Check sheet for the modelled part. Datum: model origin and axes. Units: mm. Face numbers are marked on the shaded views. A direction names the side the tool comes from. Round coordinates to 2 decimals unless told otherwise and drop trailing zeros. Loops run counter-clockwise (first coordinate to the right, second up) from the corner with the lowest first, then second, coordinate; pieces in that order, holes last. Notation, with made-up numbers: M 53,64.5 L 86,64.5 A24 ccw 86,79.5 Z; hole C 28,60 d8. An arc over 180 degrees is marked long. Write item = value, one per line. Start each with the question number.
(1) Cross-section at D-D on y = 0. Record the boundary of the cut face in (x, z), plus the area to 3 significant figures.
(2) Set-up check for the marked faces 4, 5 and 6: record each of +Z, -Z, +X, -X, +Y, -Y from which the full face is reachable in a straight line by a thin tool's end or side.
(3) Mould release check, pull along Z, two halves, no side actions. Record for the marked faces 1, 2 and 3: pulls with the +Z half, pulls with the -Z half, needs draft (parallel to the pull), parting line crosses it, or undercut.
(4) Cross-section at A-A on z = 10.75. Record the boundary of the cut face in (x, y).
(5) Cross-section at C-C on y = 6. Record the boundary of the cut face in (x, z).
(6) Scan lines: L1, parallel to Y at x = 1.45, z = -10.75; L2, parallel to X at y = -2.75, z = 13; L3, parallel to Y at x = 1, z = 0. Record each from-to range of solid material in increasing order. Write a range as from..to.
(7) Cross-section at B-B on x = 2.5. Record the boundary of the cut face in (y, z), plus the area to 3 significant figures.
(8) Go/stop test with flat-tipped pins: P1, Ø1, axis at x = 1, y = 3, coming from the +Z side; P2, Ø0.6, axis at x = 2, y = 3, coming from the -Z side; P3, Ø2, axis at y = 0, z = 10.75, coming from the +X side; P4, Ø4, axis at y = 0, z = -10.75, coming from the +X side. Record where each tip stops, or that it passes through.
from build123d import *

# Parameters (mm, degrees)
SKETCH1_W           = 40
SKETCH1_H           = 15
BOSS_EXTRUDE1_DEPTH = 3
SKETCH2_R           = 1.25
CUT_EXTRUDE1_DEPTH  = 5
FILLET1_R           = 8
BOSS_EXTRUDE2_START = 4
BOSS_EXTRUDE2_DEPTH = 4
FILLET2_R           = 4


with BuildPart() as part:
    # Sketch1 → Boss-Extrude1 (new body)
    with BuildSketch(Plane(origin=(0, 0, 0), x_dir=(0, 0, -1), z_dir=(1, 0, 0))):
        Rectangle(SKETCH1_W, SKETCH1_H)
    extrude(amount=BOSS_EXTRUDE1_DEPTH)

    # Sketch2 → Cut-Extrude1 (cut)
    with BuildSketch(Plane(origin=(3, 0, 0), x_dir=(0, 0, -1), z_dir=(1, 0, 0))):
        with Locations((-10.75, 0)):
            Circle(SKETCH2_R)
        with BuildLine():
            Line((-3, 2.25), (-3, 7.5))
            Line((-3, 7.5), (3, 7.5))
            Line((3, 7.5), (3, 2.25))
            ThreePointArc((3, 2.25), (0, -0.75), (-3, 2.25))
        make_face()
    cut_extrude1 = extrude(amount=-CUT_EXTRUDE1_DEPTH, mode=Mode.SUBTRACT)

    # Mirror1: Cut-Extrude1 across plane
    add(cut_extrude1.mirror(Plane.XY), mode=Mode.SUBTRACT)

    # Fillet1
    fillet1_edges = [part.edges().sort_by_distance(p)[0] for p in [
        (1.5, 7.5, 20),
        (1.5, 7.5, -20),
    ]]
    fillet(fillet1_edges, radius=FILLET1_R)

    # Sketch3 → Boss-Extrude2 (add)
    with BuildSketch(Plane(origin=(3, 0, 0), x_dir=(0, 0, -1), z_dir=(1, 0, 0)).offset(BOSS_EXTRUDE2_START)):
        with BuildLine():
            Line((-3, 2.25), (-5.5, 2.25))
            ThreePointArc((-5.5, 2.25), (0, -5.942432162), (5.5, 2.25))
            Line((5.5, 2.25), (3, 2.25))
            ThreePointArc((3, 2.25), (0, -0.75), (-3, 2.25))
        make_face()
    extrude(amount=-BOSS_EXTRUDE2_DEPTH)

    # Fillet2
    fillet2_edges = [part.edges().sort_by_distance(p)[0] for p in [
        (1.5, 7.5, 3),
        (1.5, 7.5, -3),
    ]]
    fillet(fillet2_edges, radius=FILLET2_R)


solid = part.part
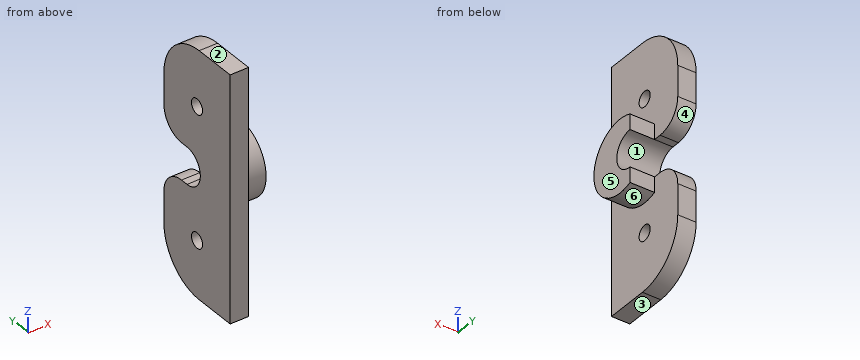
Result:
q1.outline = M 0,-19.98 L 3,-19.98 L 3,-12 L 0,-12 Z; M 0,-9.5 L 3,-9.5 L 3,-5.94 L 7,-5.94 L 7,-1.98 L 0,-1.98 Z; M 0,1.98 L 7,1.98 L 7,5.94 L 3,5.94 L 3,9.5 L 0,9.5 Z; M 0,12 L 3,12 L 3,19.98 L 0,19.98 Z
q1.area = 125 mm^2
q2.face_4 = +X, -X, +Y
q2.face_5 = +Z, -Z, +X, +Y, -Y
q2.face_6 = +X
q3.face_1 = undercut
q3.face_2 = pulls with the +Z half
q3.face_3 = pulls with the -Z half
q4.outline = M 0,-7.5 L 3,-7.5 L 3,-1.25 L 0,-1.25 Z; M 0,1.25 L 3,1.25 L 3,7.5 L 0,7.5 Z
q5.outline = M 0,-16.66 L 3,-16.66 L 3,-3.88 L 0,-3.88 Z; M 0,3.88 L 3,3.88 L 3,16.66 L 0,16.66 Z
q6.L1 = -7.5..-1.25, 1.25..7.5
q6.L2 = 0..3
q6.L3 = -7.5..-0.75
q7.outline = M -7.5,-20 L -0.5,-20 A8 ccw 7.5,-12 L 7.5,-7 A4 ccw 3.5,-3 L 2.25,-3 A3 cw 2.25,3 L 3.5,3 A4 ccw 7.5,7 L 7.5,12 A8 ccw -0.5,20 L -7.5,20 Z; hole C 0,-10.75 d2.5; hole C 0,10.75 d2.5
q7.area = 510 mm^2
q8.P1 = 19.42
q8.P2 = -19.33
q8.P3 = through
q8.P4 = 3
